```python
from build123d import *

# Parameters (mm, degrees)
BOSS_EXTRUDE1_DEPTH = 26.9875
BOSS_EXTRUDE5_START = -6.35
BOSS_EXTRUDE5_DEPTH = 6.35
SKETCH3_W           = 25.4
SKETCH3_H           = 33.3375
BOSS_EXTRUDE7_DEPTH = 45.72
SKETCH6_W           = 8.89
SKETCH6_H           = 33.3375
BOSS_EXTRUDE8_DEPTH = 22.86
SKETCH7_W           = 22.86
SKETCH7_H           = 14.5415
SKETCH7_H_2         = 6.604
CUT_EXTRUDE1_DEPTH  = 21.082
SKETCH11_W          = 51.2557102
SKETCH11_H          = 7.9375
CUT_EXTRUDE3_DEPTH  = 13.716
SHELL1_START        = 3.81
SHELL1_DEPTH        = 23.1775
SHELL1_START_2      = 25.4635
SHELL1_2_DEPTH      = 1.524
SKETCH13_R          = 1.26873
CUT_EXTRUDE4_DEPTH  = 35.56
SKETCH14_W          = 40.64
SKETCH14_H          = 6.35
BOSS_EXTRUDE9_DEPTH = 22.86
CUT_EXTRUDE5_REACH  = 156.884
SKETCH16_R          = 3.81


# Read off the part's stored shape, not the designer's step: Shell1
with BuildPart() as part:
    # Sketch1 → Boss-Extrude1 (new body)
    with BuildSketch(Plane(origin=(0, 0, 0), x_dir=(1, 0, 0), z_dir=(0, 1, 0))):
        with BuildLine():
            ThreePointArc((-27.606252307, 13.699523808), (-37.835547974, 38.395228141), (-62.531252307, 48.624523808))
            Line((-62.531252307, 48.624523808), (-62.531252307, 45.513023808))
            ThreePointArc((-62.531252307, 45.513023808), (-40.035710723, 36.195065391), (-30.717752307, 13.699523808))
            ThreePointArc((-30.717752307, 13.699523808), (-40.035710723, -8.796017775), (-62.531252307, -18.113976192))
            Line((-62.531252307, -18.113976192), (-62.531252307, -21.225476192))
            ThreePointArc((-62.531252307, -21.225476192), (-37.835547974, -10.996180525), (-27.606252307, 13.699523808))
        make_face()
        with BuildLine():
            Line((-62.531252307, 45.513023808), (-62.531252307, 48.624523808))
            ThreePointArc((-62.531252307, 48.624523808), (-68.595914912, 48.093934582), (-74.476305812, 46.518288589))
            Line((-74.476305812, 46.518288589), (-73.412110136, 43.594434999))
            ThreePointArc((-73.412110136, 43.594434999), (-68.055608607, 45.029705258), (-62.531252307, 45.513023808))
        make_face()
        with BuildLine():
            ThreePointArc((-74.476305812, -19.119240973), (-68.595914912, -20.694886966), (-62.531252307, -21.225476192))
            Line((-62.531252307, -21.225476192), (-62.531252307, -18.113976192))
            ThreePointArc((-62.531252307, -18.113976192), (-68.055608607, -17.630657643), (-73.412110136, -16.195387383))
            Line((-73.412110136, -16.195387383), (-74.476305812, -19.119240973))
        make_face()
        with BuildLine():
            Line((13.643756331, 48.624523808), (-62.531252307, 48.624523808))
            ThreePointArc((-62.531252307, 48.624523808), (-37.835547974, 38.395228141), (-27.606252307, 13.699523808))
            ThreePointArc((-27.606252307, 13.699523808), (-37.835547974, -10.996180525), (-62.531252307, -21.225476192))
            Line((-62.531252307, -21.225476192), (13.643756331, -21.225476192))
            Line((13.643756331, -21.225476192), (13.643756331, 48.624523808))
        make_face()
    boss_extrude1 = extrude(amount=BOSS_EXTRUDE1_DEPTH)

    # Sketch1<5> → Boss-Extrude5 (add)
    with BuildSketch(Plane(origin=(0, 0, 0), x_dir=(1, 0, 0), z_dir=(0, 1, 0)).offset(BOSS_EXTRUDE5_START)):
        with BuildLine():
            Line((-62.531252307, -21.225476192), (13.643756331, -21.225476192))
            Line((13.643756331, -21.225476192), (13.643756331, 48.624523808))
            Line((13.643756331, 48.624523808), (-62.531252307, 48.624523808))
            ThreePointArc((-62.531252307, 48.624523808), (-97.456252307, 13.699523808), (-62.531252307, -21.225476192))
        make_face()
    boss_extrude5 = extrude(amount=BOSS_EXTRUDE5_DEPTH)

    # Mirror1: Boss-Extrude1, Boss-Extrude5 across plane
    add(boss_extrude1.mirror(Plane(origin=(13.643756331, 26.9875, 0), x_dir=(0, 0, 1), z_dir=(1, 0, 0))))
    add(boss_extrude5.mirror(Plane(origin=(13.643756331, 26.9875, 0), x_dir=(0, 0, 1), z_dir=(1, 0, 0))))

    # Sketch3 → Boss-Extrude7 (add)
    with BuildSketch(Plane.XY.offset(21.225476192)):
        with Locations((0.943756331, 10.31875)):
            Rectangle(SKETCH3_W, SKETCH3_H)
        with Locations((26.343756331, 10.31875)):
            Rectangle(SKETCH3_W, SKETCH3_H)
    extrude(amount=BOSS_EXTRUDE7_DEPTH)

    # Sketch6 → Boss-Extrude8 (add)
    with BuildSketch(Plane.XY.offset(66.945476192)):
        with Locations((9.198756331, 10.31875)):
            Rectangle(SKETCH6_W, SKETCH6_H)
        with Locations((18.088756331, 10.31875)):
            Rectangle(SKETCH6_W, SKETCH6_H)
    extrude(amount=BOSS_EXTRUDE8_DEPTH)

    # Sketch7 → Cut-Extrude1 (cut)
    with BuildSketch(Plane.ZY.offset(-4.753756331)):
        with Locations((78.375476192, 19.71675)):
            Rectangle(SKETCH7_W, SKETCH7_H)
        with Locations((78.375476192, 3.048)):
            Rectangle(SKETCH7_W, SKETCH7_H_2)
    extrude(amount=-CUT_EXTRUDE1_DEPTH, mode=Mode.SUBTRACT)

    # Sketch11 → Cut-Extrude3 (cut)
    with BuildSketch(Plane.XY.offset(21.225476192)):
        with Locations((-52.116098769, 11.33475)):
            Rectangle(SKETCH11_W, SKETCH11_H)
    cut_extrude3 = extrude(amount=-CUT_EXTRUDE3_DEPTH, mode=Mode.SUBTRACT)

    # Mirror2: Cut-Extrude3 across plane
    add(cut_extrude3.mirror(Plane(origin=(13.64376748, 0, 0), x_dir=(0, 0, 1), z_dir=(1, 0, 0))), mode=Mode.SUBTRACT)

    # Shell1 outline → Shell1 (cut)
    with BuildSketch(Plane(origin=(0, 0, 0), x_dir=(1, 0, 0), z_dir=(0, 1, 0)).offset(SHELL1_START)):
        with BuildLine():
            Line((-16.328243669, 2.650523808), (-16.328243669, -11.065476192))
            Line((-16.328243669, -11.065476192), (-1.596243669, -11.065476192))
            Line((-1.596243669, -11.065476192), (-1.596243669, -56.785476192))
            Line((-1.596243669, -56.785476192), (28.883756331, -56.785476192))
            Line((28.883756331, -56.785476192), (28.883756331, -11.065476192))
            Line((28.883756331, -11.065476192), (43.615778629, -11.065476192))
            Line((43.615778629, -11.065476192), (43.615778629, 2.650523808))
            Line((43.615778629, 2.650523808), (49.325626028, 2.650523808))
            ThreePointArc((49.325626028, 2.650523808), (48.541178718, 21.311066068), (55.929688893, 38.464523808))
            Line((55.929688893, 38.464523808), (-28.642176231, 38.464523808))
            ThreePointArc((-28.642176231, 38.464523808), (-21.253666056, 21.311066068), (-22.038113366, 2.650523808))
            Line((-22.038113366, 2.650523808), (-16.328243669, 2.650523808))
        make_face()
    extrude(amount=SHELL1_DEPTH, mode=Mode.SUBTRACT)

    # Shell1 2 outline → Shell1 2 (cut)
    with BuildSketch(Plane(origin=(0, 0, 0), x_dir=(1, 0, 0), z_dir=(0, 1, 0)).offset(SHELL1_START_2)):
        with BuildLine():
            ThreePointArc((-22.038113366, 2.650523808), (-24.713126472, -4.509376779), (-28.642176231, -11.065476192))
            Line((-28.642176231, -11.065476192), (-16.328243669, -11.065476192))
            Line((-16.328243669, -11.065476192), (-16.328243669, 2.650523808))
            Line((-16.328243669, 2.650523808), (-22.038113366, 2.650523808))
        make_face()
        with BuildLine():
            ThreePointArc((55.929688893, -11.065476192), (52.000639133, -4.509376779), (49.325626028, 2.650523808))
            Line((49.325626028, 2.650523808), (43.615778629, 2.650523808))
            Line((43.615778629, 2.650523808), (43.615778629, -11.065476192))
            Line((43.615778629, -11.065476192), (55.929688893, -11.065476192))
        make_face()
    extrude(amount=SHELL1_2_DEPTH, mode=Mode.SUBTRACT)

    # Sketch13 → Cut-Extrude4 (cut)
    with BuildSketch(Plane(origin=(0, 26.9875, 0), x_dir=(1, 0, 0), z_dir=(0, 1, 0))):
        with Locations(Location((33.963756331, -16.145476192, 0), (0, 0, 270))):
            Circle(SKETCH13_R)
        with Locations(Location((-6.676243669, -16.145476192, 0), (0, 0, 270))):
            Circle(SKETCH13_R)
        with Locations(Location((-6.676243669, 43.544523808, 0), (0, 0, 270))):
            Circle(SKETCH13_R)
        with Locations(Location((33.963756331, 43.544523808, 0), (0, 0, 270))):
            Circle(SKETCH13_R)
    extrude(amount=-CUT_EXTRUDE4_DEPTH, mode=Mode.SUBTRACT)

    # Sketch14 → Boss-Extrude9 (add)
    with BuildSketch(Plane.XY.offset(66.945476192)):
        with Locations((13.64376748, 9.525)):
            Rectangle(SKETCH14_W, SKETCH14_H)
        with Locations((13.64376748, -3.175)):
            Rectangle(SKETCH14_W, SKETCH14_H)
    extrude(amount=BOSS_EXTRUDE9_DEPTH)

    # Cut-Extrude5: up to this face of the body (flat: up to its plane)
    cut_extrude5_end = Plane(part.part.faces().sort_by_distance((13.643756916, -6.35, -1.287747725))[0])
    # Sketch16 → Cut-Extrude5 (cut, up to the picked face)
    with BuildSketch(Plane(origin=(0, 12.7, 0), x_dir=(1, 0, 0), z_dir=(0, 1, 0)), mode=Mode.PRIVATE) as cut_extrude5_sk1:
        with Locations(Location((3.48376748, -78.375476192, 0), (0, 0, 270))):
            Circle(SKETCH16_R)
    cut_extrude5_tool1 = split(extrude(cut_extrude5_sk1.sketch, amount=-CUT_EXTRUDE5_REACH, mode=Mode.PRIVATE), bisect_by=cut_extrude5_end, keep=Keep.BOTH, mode=Mode.PRIVATE)
    cut_extrude5 = cut_extrude5_tool1.solids().sort_by(Axis((3.483767, 12.7, 78.375476), (0, -1, 0)))[0]
    add(cut_extrude5, mode=Mode.SUBTRACT)

    # Mirror3: Cut-Extrude5 across plane
    add(cut_extrude5.mirror(Plane(origin=(13.64376748, 0, 0), x_dir=(0, 0, 1), z_dir=(1, 0, 0))), mode=Mode.SUBTRACT)


solid = part.part
```
For this review, take the finished solid that the model builds, in its own axes (mm). A direction names the side the tool comes from. Give positions to 0.01 mm unless a question says otherwise; leave off trailing zeros. Order: outer loops, then holes, each group sorted by start corner. A loop starts at its lowest first (then second) coordinate and runs counter-clockwise, first axis right, second up.
1) Insertion check: pin 1 (2 mm diameter, centred on x = -6.68, z = -43.54, fed in from -Y); pin 2 (10 mm diameter, centred on x = 22.5, z = 45.5, fed in from +Y); pin 3 (3 mm diameter, centred on y = -3.5, z = 76, fed in from +X); pin 4 (2.5 mm diameter, centred on x = 60, y = 12, fed in from +Z). Each pin has a flat end and moves straight along its axis. Give the tip position at first contact, or say it passes through.
2) Take a section at B-B (z = 24). Give the boundary of the cut face in (x, y), then the cut area to 3 significant figures.
3) The part is to be moulded in two halves that separate along Z. For faces 6 (the face through (43.616, 14, 4)), 7 (the face through (13, 10, -48.625)), 8 (the face through (92, 0, -14)), 9 (the face through (95.97, 21.06, 20.68)), say which applies: released by +Z, released by -Z, zero draft, split by the parting line, or undercut.
4) Wall thickness on line 1 (X direction, y = 7, z = 53.5); line 2 (Z direction, x = 36, y = 13.5); line 3 (Y direction, x = -49, z = -37): over which ranges is each line inside the solid? List them lowest first.
5) Take a section at C-C (y = 19.5). State how many separate pieces and enclosed holes the cut face has, then the cut area to 3 significant figures.
6) Take a section at D-D (z = -29). Give the boundary of the cut face in (x, y), then the cut area to 3 significant figures.
7) Take a section at A-A (x = 71.5). Give the boundary of the cut face in (y, z), then the cut area to 3 significant figures.
8) For faces 1 (the face through (13, 12.7, 78)), 2 (the face through (13, 6.35, 78)), 3 (the face through (13, 15, 56.785)), 4 (the face through (-6.676, -3, 78)), 5 (the face through (39.044, 10, 44)), list the 3-axis set-ups (+Z, -Z, +X, -X, +Y, -Y) from which the entire face can be reached by the end or side of a thin tool; tool diameter is ignored.
Derived:
1. pin 1: passes through
1. pin 2: stops at y = 3.81
1. pin 3: stops at x = 33.96
1. pin 4: stops at z = 7.51
2. outline: (-11.76, -6.35) - (39.04, -6.35) - (39.04, 26.99) - (28.88, 26.99) - (28.88, 3.81) - (-1.6, 3.81) - (-1.6, 26.99) - (-11.76, 26.99) - close
2. area: 987 mm2
3. face 6: undercut
3. face 7: released by -Z
3. face 8: undercut
3. face 9: released by +Z
4. line 1: x = -11.76 to -1.6, 28.88 to 39.04
4. line 2: z = -48.62 to -38.46, 11.07 to 66.95
4. line 3: y = -6.35 to 0
5. separate pieces: 1
5. enclosed holes: 5
5. area: 5,110 mm2
6. outline: (-93.93, -6.35) - (121.21, -6.35) - (121.21, 0) - (61.93, 0) - (61.93, 26.99) - (50.73, 26.99) - (50.73, 3.81) - (-23.45, 3.81) - (-23.45, 26.99) - (-34.64, 26.99) - (-34.64, 0) - (-93.93, 0) - close
6. area: 2,250 mm2
7. outline: (-6.35, -48.62) - (26.99, -48.62) - (26.99, -39.71) - (0, -39.71) - (0, 12.31) - (7.37, 12.31) - (7.37, 21.23) - (-6.35, 21.23) - close; (15.3, 12.31) - (26.99, 12.31) - (26.99, 21.23) - (15.3, 21.23) - close
7. area: 854 mm2
8. face 1: +Z, +X, -X, +Y
8. face 2: +Z, +X, -X
8. face 3: +Y
8. face 4: +Z, -X, +Y, -Y
8. face 5: +Z, +X, +Y, -Y
